Could you check a few things on this drawing? It's one solid part, dimensions in mm from its lowest x, y, z. A direction names the side the tool comes from. Round coordinates to 2 decimals unless told otherwise and drop trailing zeros. Write each loop counter-clockwise with the first axis right and the second up, starting at its lowest first coordinate (ties: lowest second). Pieces come first, ordered by that corner, then holes. Notation, with made-up numbers: M 57.5,1 L 78.5,1 A22 ccw 78.5,17 Z; hole C 15.25,-12.75 d9. An arc over 180 degrees is marked long. One line per question, with ' | ' between items. Start each with the question number.
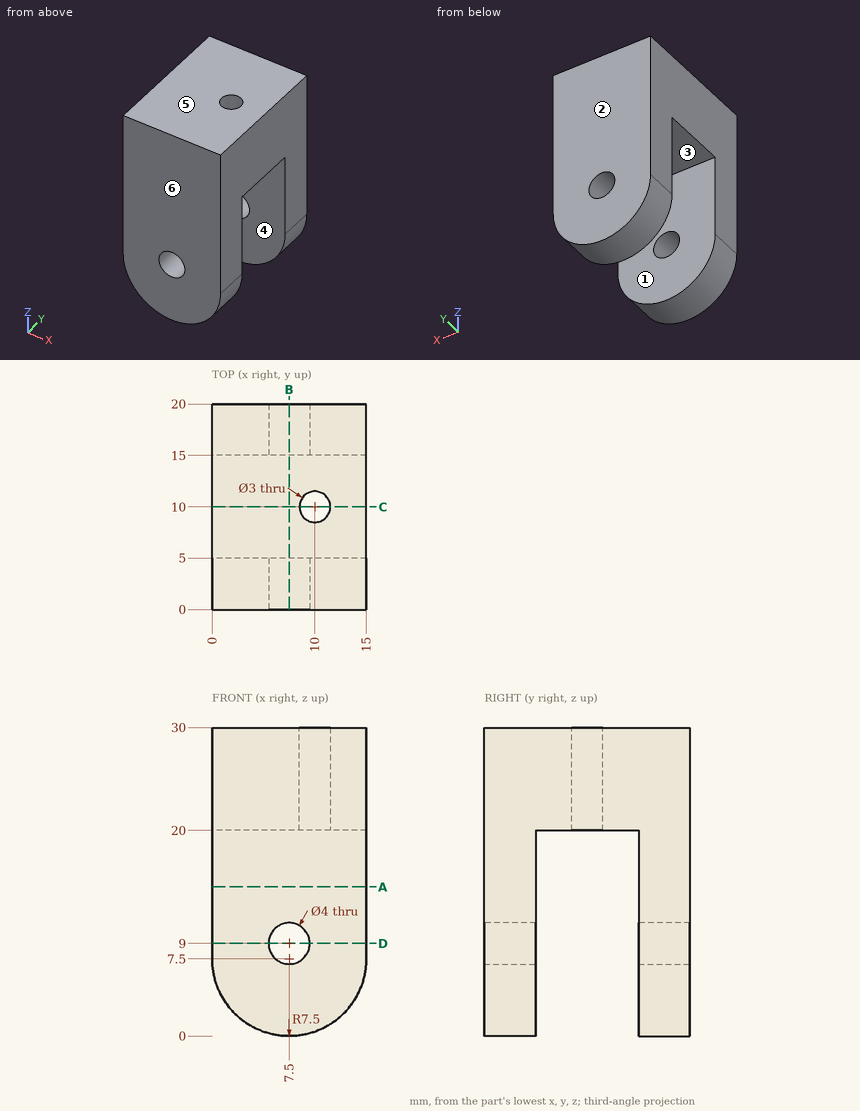
1. I'm going to push a flat-ended pin straight in: P1, Ø4, axis at x = 12, y = 12, coming from the -Z side. Where does the tip first touch, or does it pass through?
2. If we mould it in two halves opening along Y, with no side actions, what happens to the marked faces 3, 4, 5 and 6? For each: released by +Y, released by -Y, zero draft, split by the parting line, or undercut.
3. I need wall thicknesses on line 1 along X through (y, z) = (16.9, 9); line 2 along Y through (x, z) = (10, 24.25); line 3 along Y through (x, z) = (9.5, 18.75). Which ranges of each line are inside material? Lowest first, please. Write a range as from..to.
4. Suppose I cut it at C-C (y = 10). Write out the boundary of the cut face in (x, z), and give its area (3 significant figures).
5. Suppose I cut it at A-A (z = 14.5). Write out the boundary of the cut face in (x, y).
6. Suppose I cut it at D-D (z = 9). Write out the boundary of the cut face in (x, y), and give its area (3 significant figures).
7. Which directions (+Z, -Z, +X, -X, +Y, -Y) give clear straight access to the entire face, cutting with the end or side of a thin tool? Please do the marked faces 1 and 2.
8. Suppose I cut it at B-B (x = 7.5). Write out the boundary of the cut face in (y, z).
Computed:
1) P1: stops at z = 20
2) face 3: undercut | face 4: undercut | face 5: zero draft | face 6: released by -Y
3) line 1: x = 0..5.5, 9.5..15 | line 2: y = 0..8.5, 11.5..20 | line 3: y = 0..5, 15..20
4) outline: M 0,20 L 8.5,20 L 8.5,30 L 0,30 Z; M 11.5,20 L 15,20 L 15,30 L 11.5,30 Z | area: 120 mm²
5) outline: M 0,0 L 15,0 L 15,5 L 0,5 Z; M 0,15 L 15,15 L 15,20 L 0,20 Z
6) outline: M 0,0 L 5.5,0 L 5.5,5 L 0,5 Z; M 0,15 L 5.5,15 L 5.5,20 L 0,20 Z; M 9.5,0 L 15,0 L 15,5 L 9.5,5 Z; M 9.5,15 L 15,15 L 15,20 L 9.5,20 Z | area: 110 mm²
7) face 1: -Z, +X, -X | face 2: +Z, -Z, +X, -X, +Y
8) outline: M 0,0 L 5,0 L 5,7 L 0,7 Z; M 0,11 L 5,11 L 5,20 L 15,20 L 15,11 L 20,11 L 20,30 L 0,30 Z; M 15,0 L 20,0 L 20,7 L 15,7 Z
